from build123d import *

# Parameters (mm, degrees)
SKETCH1_W           = 29.5
SKETCH1_H           = 10
SKETCH1_H_2         = 8
SKETCH1_R           = 1.65
BOSS_EXTRUDE1_DEPTH = 6
SKETCH3_W           = 29.5
SKETCH3_H           = 7
BOSS_EXTRUDE3_DEPTH = 11


with BuildPart() as part:
    # Sketch1 → Boss-Extrude1 (new body)
    # profile 1 of 2: a face of its own
    with BuildSketch(Plane(origin=(0, 0, 0), x_dir=(1, 0, 0), z_dir=(0, 1, 0))):
        with Locations((0, 9)):
            Rectangle(SKETCH1_W, SKETCH1_H)
    # profile 2 of 2: a face of its own
    with BuildSketch(Plane(origin=(0, 0, 0), x_dir=(1, 0, 0), z_dir=(0, 1, 0))):
        Rectangle(SKETCH1_W, SKETCH1_H_2)
        with Locations(Location((0, 0.7, 0), (0, 0, 270))):
            Circle(SKETCH1_R, mode=Mode.SUBTRACT)
    extrude(amount=BOSS_EXTRUDE1_DEPTH)

    # Sketch3 → Boss-Extrude3 (add)
    with BuildSketch(Plane(origin=(0, 6, 0), x_dir=(1, 0, 0), z_dir=(0, 1, 0))):
        with Locations((0, 10.5)):
            Rectangle(SKETCH3_W, SKETCH3_H)
    extrude(amount=BOSS_EXTRUDE3_DEPTH)


solid = part.part
Part model, mm, in its own coordinate system. Give positions to 0.01 mm unless a question says otherwise; leave off trailing zeros. Loops run counter-clockwise (first coordinate to the right, second up) from the corner with the lowest first, then second, coordinate; pieces in that order, holes last.
(1) Pin check, flat tips, straight feed: pin 1 (8 mm diameter, centred on x = -9.5, z = 0.5, fed in from +Y); pin 2 (8 mm diameter, centred on x = 1.5, y = 12.5, fed in from +Z). Stop position of each tip, or through.
Return value:
pin 1: stops at y = 6
pin 2: stops at z = -7
(2) Band-saw the part on A-A (z = -0.7). Write the cut outline in (x, y).
Return value:
outline: (-14.75, 0) - (-1.65, 0) - (-1.65, 6) - (-14.75, 6) - close; (1.65, 0) - (14.75, 0) - (14.75, 6) - (1.65, 6) - close
(3) Band-saw the part on C-C (y = 4.5). Write the cut outline in (x, z).
Return value:
outline: (-14.75, -14) - (14.75, -14) - (14.75, 4) - (-14.75, 4) - close; hole circle Ø3.3 at (0, -0.7)
(4) Band-saw the part on D-D (x = 5). Write the cut outline in (y, z).
Return value:
outline: (0, -14) - (17, -14) - (17, -7) - (6, -7) - (6, 4) - (0, 4) - close
(5) Drill centre lines: line 1 along X through (y, z) = (4.5, -0.7); line 2 along Z through (x, y) = (5.5, 14.25); line 3 along Y through (x, z) = (-6.75, -6.75). Where is each one in solid material? Low to high.
Return value:
line 1: x = -14.75 to -1.65, 1.65 to 14.75
line 2: z = -14 to -7
line 3: y = 0 to 6
(6) Band-saw the part on B-B (x = 0). Write the cut outline in (y, z).
Return value:
outline: (0, -14) - (17, -14) - (17, -7) - (6, -7) - (6, -2.35) - (0, -2.35) - close; (0, 0.95) - (6, 0.95) - (6, 4) - (0, 4) - close
(7) Pull direction Z, two halves, no side cores. Call faces 1 (the flat face through (0, 6, -3)), 2 (the flat face through (0, 11, -7)), 3 (the flat face through (0, 8, -14)), 4 (the cylindrical face through (-0.632, 2.958, 0.824)): pulls with the +Z half, pulls with the -Z half, needs draft (parallel to the pull), parting line crosses it, or undercut.
Return value:
face 1: needs draft
face 2: pulls with the +Z half
face 3: pulls with the -Z half
face 4: undercut
